Source: CAD feature listing. Evaluate the final solid. Frame: model axes, mm. Give positions to 0.01 mm unless a question says otherwise; leave off trailing zeros. Loops run counter-clockwise (first coordinate to the right, second up) from the corner with the lowest first, then second, coordinate; pieces in that order, holes last.
```python
from build123d import *

# Parameters (mm, degrees)
F0_R     = 2.5
F1_DEPTH = 8
F2_R     = 4


with BuildPart() as f1:
    # F0 (on Top) → F1 (new body)
    with BuildSketch(Plane.XY):
        with BuildLine():
            Line((-21, 21), (-21, 16))
            Line((-21, 16), (-18.5, 16))
            ThreePointArc((-18.5, 16), (-17.767767, 17.767767), (-16, 18.5))
            Line((-16, 18.5), (-16, 21))
            Line((-16, 21), (-21, 21))
        make_face()
        with BuildLine():
            Line((-21, -21), (21, -21))
            Line((21, -21), (21, 21))
            Line((21, 21), (-16, 21))
            Line((-16, 21), (-16, 18.5))
            ThreePointArc((-16, 18.5), (-14.232233, 17.767767), (-13.5, 16))
            ThreePointArc((-13.5, 16), (-16, 13.5), (-18.5, 16))
            Line((-18.5, 16), (-21, 16))
            Line((-21, 16), (-21, -21))
        make_face()
        with Locations((-16, -16)):
            Circle(F0_R, mode=Mode.SUBTRACT)
        with Locations((16, -16)):
            Circle(F0_R, mode=Mode.SUBTRACT)
        with Locations((16, 16)):
            Circle(F0_R, mode=Mode.SUBTRACT)
    extrude(amount=F1_DEPTH)

    # F2
    f2_edges = [f1.edges().sort_by_distance(p)[0] for p in [
        (21, -21, 4),
        (-21, -21, 4),
        (21, 21, 4),
        (-21, 21, 4),
    ]]
    fillet(f2_edges, radius=F2_R)


solid = f1.part
```
(1) Ray query, line 1 along Y through (x, z) = (16, 5.25); line 2 along X through (y, z) = (-14.5, 7); line 3 along Y through (x, z) = (-17.5, 6). Return the intervals inside material, ascending.
A:
line 1: y = -21 to -18.5, -13.5 to 13.5, 18.5 to 21
line 2: x = -21 to -18, -14 to 14, 18 to 21
line 3: y = -20.97 to -18, -14 to 14, 18 to 20.97
(2) Section C-C, the plane z = 6.5. Return the cut outline in (x, y).
A:
outline: (-21, -17) arc R4 ccw to (-17, -21) - (17, -21) arc R4 ccw to (21, -17) - (21, 17) arc R4 ccw to (17, 21) - (-17, 21) arc R4 ccw to (-21, 17) - close; hole circle Ø5 at (-16, -16); hole circle Ø5 at (-16, 16); hole circle Ø5 at (16, -16); hole circle Ø5 at (16, 16)
(3) First-contact query: pin 1 (4 mm diameter, centred on x = 16, y = 16, fed in from -Z). Flat tip, straight axial feed; report the tip coordinate or a pass-through.
A:
pin 1: passes through
(4) Mould query, pull axis X, two halves, no side actions, for faces 1 (the flat face through (0, -21, 4)), 2 (the cylindrical face through (-19.859, 19.797, 4.056)), 3 (the cylindrical face through (13.5, -15.9, 3.9)). Classes: pulls with the +X half, pulls with the -X half, needs draft (parallel to the pull), parting line crosses it, or undercut.
A:
face 1: needs draft
face 2: pulls with the -X half
face 3: undercut
(5) Section A-A, the plane x = 16. Return the cut outline in (y, z), then the cut area to 3 significant figures.
A:
outline: (-21, 0) - (-18.5, 0) - (-18.5, 8) - (-21, 8) - close; (-13.5, 0) - (13.5, 0) - (13.5, 8) - (-13.5, 8) - close; (18.5, 0) - (21, 0) - (21, 8) - (18.5, 8) - close
area: 256 mm2
